Work out the finished part from the listing and answer in its coordinate system (mm). A direction names the side the tool comes from. Coordinates: 2 decimals unless noted, no trailing zeros. Use a Markdown table: item, result.
from build123d import *

# Parameters (mm, degrees)
SKETCH3_R          = 1.5
CUT_EXTRUDE1_DEPTH = 7


with BuildPart() as part:
    # Sketch2 → Loft1 section 0
    with BuildSketch(Plane(origin=(0, -10, 0), x_dir=(1, 0, 0), z_dir=(0, 1, 0))):
        with BuildLine():
            Line((6.413648207, 14.153454805), (-7.066772303, 13.838926817))
            Line((-7.066772303, 13.838926817), (-15.225769132, 3.103404673))
            Line((-15.225769132, 3.103404673), (-11.919451256, -9.969044488))
            Line((-11.919451256, -9.969044488), (0.362456529, -15.534599818))
            Line((0.362456529, -15.534599818), (12.371427154, -9.402284637))
            Line((12.371427154, -9.402284637), (15.064460802, 3.810142647))
            Line((15.064460802, 3.810142647), (6.413648207, 14.153454805))
        make_face()
    # Sketch1 → Loft1 section 1
    with BuildSketch(Plane(origin=(0, 0, 0), x_dir=(1, 0, 0), z_dir=(0, 1, 0))):
        with BuildLine():
            Line((7.953060314, -6.044325838), (9.68429623, 2.449377416))
            Line((9.68429623, 2.449377416), (4.123059561, 9.098649518))
            Line((4.123059561, 9.098649518), (-4.542925052, 8.896452954))
            Line((-4.542925052, 8.896452954), (-9.787994442, 1.995045862))
            Line((-9.787994442, 1.995045862), (-7.662504379, -6.408671456))
            Line((-7.662504379, -6.408671456), (0.233007768, -9.986528454))
            Line((0.233007768, -9.986528454), (7.953060314, -6.044325838))
        make_face()
    loft()

    # Sketch3 → Cut-Extrude1 (cut)
    with BuildSketch(Plane.XZ.offset(10)):
        with Locations(Location((0, 0, 0), (0, 0, 270))):
            Circle(SKETCH3_R)
    extrude(amount=-CUT_EXTRUDE1_DEPTH, mode=Mode.SUBTRACT)


solid = part.part
Q1. Determine the mould class of faces 1 (the cylindrical face through (0.45, -6.55, -1.43)), 2 (the flat face through (-1, 0, 0)) for opening direction Z: pulls with the +Z half, pulls with the -Z half, needs draft (parallel to the pull), parting line crosses it, or undercut.
Solved:
| item | result |
|---|---|
| face 1 | undercut |
| face 2 | needs draft |
Q2. Given pin 1 Ø0.9 at (x, z) = (-0.5, -0.5) entering from -Y; pin 2 Ø5 at (y, z) = (-1.5, 6.5) entering from +X; pin 3 Ø2 at (x, y) = (7, -2) entering from -Z, each flat-ended and moving along its own axis, determine where each tip first touches the part or whether it passes through.
Solved:
| item | result |
|---|---|
| pin 1 | y = -3 |
| pin 2 | x = 10 |
| pin 3 | z = -8.64 |
Q3. Consider line 1 (X direction, y = -5.75, z = 0); line 2 (X direction, y = -6.75, z = 0); line 3 (Y direction, x = 0, z = 13). Determine where each line is inside the solid, lowest interval first. Write a range as [from, to].
Solved:
| item | result |
|---|---|
| line 1 | [-12.25, -1.5], [1.5, 12.12] |
| line 2 | [-12.76, -1.5], [1.5, 12.63] |
| line 3 | [-10, -5.68] |
Q4. For faces 3 (the flat face through (0, -3, 0)), 4 (the flat face through (-2, -10, -2)), determine the directions among +Z, -Z, +X, -X, +Y, -Y from which every point of the face is accessible in a straight line to the end or side of a thin tool.
Solved:
| item | result |
|---|---|
| face 3 | -Y |
| face 4 | +Z, -Z, +X, -X, -Y |
